Geometry: final body of the model. Coordinates: model frame, mm. A direction names the side the tool comes from. Give positions to 0.01 mm unless a question says otherwise; leave off trailing zeros. Write each loop counter-clockwise with the first axis right and the second up, starting at its lowest first coordinate (ties: lowest second). Pieces come first, ordered by that corner, then holes. Notation, with made-up numbers: M 84.25,31.25 L 120.25,31.25 A24 cw 120.25,51.25 Z; hole C 27.5,-30 d1. An arc over 180 degrees is marked long. Use a Markdown table: item, result. Add a question column.
(1) Cut plane C-C (x = -56). Output: boundary loops of the cut face in (y, z), plus the area to 3 significant figures.
(2) Draft query along Y for faces 6 (the flat face through (-85, 14.925, 3)), 7 (the flat face through (-59, 67.925, 3)), 8 (the flat face through (-67, 45, 5)). Return one class per face: released by +Y, released by -Y, zero draft, split by the parting line, or undercut.
(3) Cut plane B-B (x = -72.5). Output: boundary loops of the cut face in (y, z), plus the area to 3 significant figures.
(4) Pin query (flat end, axial travel): pin 1 Ø1.5 at (x, z) = (-81, 2.5) entering from +Y; pin 2 Ø1.5 at (x, z) = (-79.5, 3) entering from -Y; pin 3 Ø0.9 at (x, z) = (-57, 2.5) entering from +Y. Return the tip coordinate at first contact, or that it passes through.
(5) Cut plane A-A (y = 21). Output: boundary loops of the cut face in (x, z).
(6) Material intervals for L1, parallel to Y at x = -75, z = 3.1; L2, parallel to X at y = 65.5, z = 1.1; L3, parallel to X at y = 18, z = 4.25, sorted ascending.
(7) Reachability of faces 1 (the flat face through (-77, 63.925, 3)), 2 (the flat face through (-80.137, 23, 3)), 3 (the flat face through (-85, 74.925, 3)), 4 (the flat face through (-87.137, 45, 3)), 5 (the flat face through (-60, 19.925, 3)) from +Z, -Z, +X, -X, +Y, -Y: full face, straight path, thin tool, end or side. Return the list, or none.
```python
from build123d import *

# Parameters (mm, degrees)
SKETCH1_W           = 40
SKETCH1_H           = 55
BOSS_EXTRUDE1_DEPTH = 5
SKETCH2_OUTSIDE_W   = 55.638
SKETCH2_OUTSIDE_H   = 70.638
CUT_EXTRUDE1_DEPTH  = 10
SKETCH2_3_W         = 5.25
SKETCH2_3_H         = 5
SKETCH2_3_W_2       = 9.5
BOSS_EXTRUDE2_DEPTH = 5


with BuildPart() as part:
    # Sketch1 → Boss-Extrude1 (new body)
    with BuildSketch(Plane.XY):
        with Locations((-67.136843489, 42.42527276)):
            Rectangle(SKETCH1_W, SKETCH1_H)
    extrude(amount=BOSS_EXTRUDE1_DEPTH)

    # Sketch2 outside → Cut-Extrude1 (cut)
    with BuildSketch(Plane.XY.offset(5)):
        with Locations((-67.137, 42.425)):
            Rectangle(SKETCH2_OUTSIDE_W, SKETCH2_OUTSIDE_H)
        Polygon((-75.886843489, 63.92527276), (-78.886843489, 63.92527276), (-78.886843489, 65.92527276), (-80.136843489, 65.92527276), (-80.136843489, 67.92527276), (-78.886843489, 67.92527276), (-78.886843489, 69.92527276), (-81.886843489, 69.92527276), (-87.136843489, 69.92527276), (-87.136843489, 14.92527276), (-47.136843489, 14.92527276), (-47.136843489, 69.92527276), (-52.386843489, 69.92527276), (-55.386843489, 69.92527276), (-55.386843489, 67.92527276), (-54.136843489, 67.92527276), (-54.136843489, 65.92527276), (-55.386843489, 65.92527276), (-55.386843489, 63.92527276), (-58.386843489, 63.92527276), (-58.386843489, 65.92527276), (-59.636843489, 65.92527276), (-59.636843489, 67.92527276), (-58.386843489, 67.92527276), (-58.386843489, 69.92527276), (-62.386843489, 69.92527276), (-71.886843489, 69.92527276), (-75.886843489, 69.92527276), (-75.886843489, 67.92527276), (-74.636843489, 67.92527276), (-74.636843489, 65.92527276), (-75.886843489, 65.92527276), align=None, mode=Mode.SUBTRACT)
    cut_extrude1 = extrude(amount=-CUT_EXTRUDE1_DEPTH, mode=Mode.SUBTRACT)

    # Sketch2<3> → Boss-Extrude2 (add)
    with BuildSketch(Plane.XY.offset(5)):
        with Locations((-84.511843489, 72.42527276)):
            Rectangle(SKETCH2_3_W, SKETCH2_3_H)
        with Locations((-67.136843489, 72.42527276)):
            Rectangle(SKETCH2_3_W_2, SKETCH2_3_H)
        with Locations((-49.761843489, 72.42527276)):
            Rectangle(SKETCH2_3_W, SKETCH2_3_H)
    boss_extrude2 = extrude(amount=-BOSS_EXTRUDE2_DEPTH)

    # Mirror1: Cut-Extrude1, Boss-Extrude2 across plane
    add(cut_extrude1.mirror(Plane.ZX.offset(44.92527276)), mode=Mode.SUBTRACT)
    add(boss_extrude2.mirror(Plane.ZX.offset(44.92527276)))


solid = part.part
```
Answer list:
| question | item | result |
|---|---|---|
| 1 | outline | M 25.93,0 L 63.93,0 L 63.93,5 L 25.93,5 Z |
| 1 | area | 190 mm² |
| 2 | face 6 | released by -Y |
| 2 | face 7 | undercut |
| 2 | face 8 | zero draft |
| 3 | outline | M 19.93,0 L 69.93,0 L 69.93,5 L 19.93,5 Z |
| 3 | area | 250 mm² |
| 4 | pin 1 | y = 69.93 |
| 4 | pin 2 | y = 19.93 |
| 4 | pin 3 | y = 63.93 |
| 5 | outline | M -87.14,0 L -78.89,0 L -78.89,5 L -87.14,5 Z; M -75.89,0 L -58.39,0 L -58.39,5 L -75.89,5 Z; M -55.39,0 L -47.14,0 L -47.14,5 L -55.39,5 Z |
| 6 | L1 | 19.93 to 21.93, 23.93 to 65.93, 67.93 to 69.93 |
| 6 | L2 | -87.14 to -78.89, -75.89 to -58.39, -55.39 to -47.14 |
| 6 | L3 | -87.14 to -81.89, -71.89 to -62.39, -52.39 to -47.14 |
| 7 | face 1 | +Z, -Z, +Y |
| 7 | face 2 | +Z, -Z |
| 7 | face 3 | +Z, -Z, +X, -X, +Y |
| 7 | face 4 | +Z, -Z, -X, +Y, -Y |
| 7 | face 5 | +Z, -Z, -Y |
